from build123d import *

# Parameters (mm, degrees)
SKETCH1_R       = 15
SKETCH1_R_2     = 1.5
SKETCH1_R_3     = 1.65
MAIN_BODY_DEPTH = 3
FILLET_2_R      = 2.54


with BuildPart() as part:
    # Sketch1 → Main Body (new body)
    with BuildSketch(Plane(origin=(0, 0, 0), x_dir=(1, 0, 0), z_dir=(0, 1, 0))):
        Polygon((22.5, -22.5), (57.5, -22.5), (57.5, -15.5), (37.5, -15.5), (37.5, 4.5), (22.5, 4.5), (22.5, 22.5), (-22.5, 22.5), (-22.5, -22.5), align=None)
        with Locations(Location((0, 0, 0), (0, 0, 270))):
            Circle(SKETCH1_R, mode=Mode.SUBTRACT)
        with Locations(Location((15.5, 15.5, 0), (0, 0, 270))):
            Circle(SKETCH1_R_2, mode=Mode.SUBTRACT)
        with Locations(Location((15.5, -15.5, 0), (0, 0, 270))):
            Circle(SKETCH1_R_2, mode=Mode.SUBTRACT)
        with Locations(Location((-15.5, -15.5, 0), (0, 0, 270))):
            Circle(SKETCH1_R_2, mode=Mode.SUBTRACT)
        with Locations(Location((-15.5, 15.5, 0), (0, 0, 270))):
            Circle(SKETCH1_R_2, mode=Mode.SUBTRACT)
        with Locations(Location((31, 0, 0), (0, 0, 270))):
            Circle(SKETCH1_R_3, mode=Mode.SUBTRACT)
        with Locations(Location((31, -19, 0), (0, 0, 270))):
            Circle(SKETCH1_R_3, mode=Mode.SUBTRACT)
        with Locations(Location((40, -19, 0), (0, 0, 270))):
            Circle(SKETCH1_R_3, mode=Mode.SUBTRACT)
        with Locations(Location((52, -19, 0), (0, 0, 270))):
            Circle(SKETCH1_R_3, mode=Mode.SUBTRACT)
    extrude(amount=MAIN_BODY_DEPTH)

    # FIllet 2
    fillet_2_edges = [part.edges().sort_by_distance(p)[0] for p in [
        (37.5, 1.5, -4.5),
        (57.5, 1.5, 15.5),
        (57.5, 1.5, 22.5),
        (-22.5, 1.5, 22.5),
        (-22.5, 1.5, -22.5),
        (22.5, 1.5, -22.5),
    ]]
    fillet(fillet_2_edges, radius=FILLET_2_R)


solid = part.part
Source: CAD feature listing. Evaluate the final solid. Frame: model axes, mm. A direction names the side the tool comes from. Give positions to 0.01 mm unless a question says otherwise; leave off trailing zeros. Write each loop counter-clockwise with the first axis right and the second up, starting at its lowest first coordinate (ties: lowest second). Pieces come first, ordered by that corner, then holes. Notation, with made-up numbers: (-14, 89.5) -> (22, 89.5) arc R29 ccw to (22, 112.5) -> close; hole circle Ø4 at (41.25, 48.5). An arc over 180 degrees is marked (long way). Write item = value, one per line.
Q1. Reachability of faces 1 (the face through (29, 1, -4.5)), 2 (the face through (0, 1, -22.5)) from +Z, -Z, +X, -X, +Y, -Y: full face, straight path, thin tool, end or side. Return the list, or none.
Here are the results:
face_1 = -Z, +X, +Y, -Y
face_2 = -Z, +X, -X, +Y, -Y
Q2. Cut plane C-C on z = 19. Return loops of the section in (x, y), then the cut area to 3 significant figures.
Here are the results:
outline = (-22.5, 0) -> (29.35, 0) -> (29.35, 3) -> (-22.5, 3) -> close; (32.65, 0) -> (38.35, 0) -> (38.35, 3) -> (32.65, 3) -> close; (41.65, 0) -> (50.35, 0) -> (50.35, 3) -> (41.65, 3) -> close; (53.65, 0) -> (57.5, 0) -> (57.5, 3) -> (53.65, 3) -> close
area = 210 mm²
Q3. Cut plane D-D on y = 0.7. State how many separate pieces and enclosed holes the cut face has, then the cut area to 3 significant figures.
Here are the results:
separate_pieces = 1
enclosed_holes = 9
area = 1,790 mm²
Q4. First-contact query: pin 1 (1.5 mm diameter, centred on y = 2, z = -14, fed in from +X); pin 2 (1.5 mm diameter, centred on x = 26.5, y = 1, fed in from -Z). Flat tips, straight axial feed; report the tip coordinate or a pass-through.
Here are the results:
pin_1 = 22.5
pin_2 = -4.5
Q5. Cut plane A-A on z = -9. Return loops of the section in (x, y).
Here are the results:
outline = (-22.5, 0) -> (-12, 0) -> (-12, 3) -> (-22.5, 3) -> close; (12, 0) -> (22.5, 0) -> (22.5, 3) -> (12, 3) -> close
Q6. Cut plane B-B on x = 31. Return loops of the section in (y, z).
Here are the results:
outline = (0, -4.5) -> (3, -4.5) -> (3, -1.65) -> (0, -1.65) -> close; (0, 1.65) -> (3, 1.65) -> (3, 17.35) -> (0, 17.35) -> close; (0, 20.65) -> (3, 20.65) -> (3, 22.5) -> (0, 22.5) -> close
Q7. Mould query, pull axis Z, two halves, no side actions, for faces 3 (the face through (17, 0, 5)), 4 (the face through (46, 1, 15.5)), 5 (the face through (-21.736, 1.521, 21.776)), 6 (the face through (-15.43, 1.48, 14)). Classes: +Z half, -Z half, draft (parallel to the pull), parting line (faces both ways), or undercut.
Here are the results:
face_3 = draft
face_4 = -Z half
face_5 = +Z half
face_6 = undercut
Q8. Line query: line 1 (X direction, y = 1.05, z = 19); line 2 (X direction, y = 1.6, z = -15.5); line 3 (X direction, y = 2.7, z = 0). Output: solid intervals per line, ascending. Write a range as from..to.
Here are the results:
line_1 = -22.5..29.35, 32.65..38.35, 41.65..50.35, 53.65..57.5
line_2 = -22.5..-17, -14..14, 17..22.5
line_3 = -22.5..-15, 15..29.35, 32.65..37.5
